```python
from build123d import *

# Parameters (mm, degrees)
SKETCH1_W            = 50.8
SKETCH1_H            = 142.24
BOSS_EXTRUDE1_DEPTH  = 38.1
SKETCH8_R            = 21.43125
BOSS_EXTRUDE2_DEPTH  = 2.54
SKETCH8_5_R          = 21.43125
BOSS_EXTRUDE9_DEPTH  = 12.7
SKETCH19_W           = 12.7
SKETCH19_H           = 6.35
BOSS_EXTRUDE10_DEPTH = 6.35
BOSS_EXTRUDE11_DEPTH = 6.35
SKETCH23_R           = 3.175
BOSS_EXTRUDE12_DEPTH = 25.4
MIRROR2_COPY_1_DEPTH = 6.35


with BuildPart() as part:
    # Sketch1 → Boss-Extrude1 (new body)
    with BuildSketch(Plane.XY):
        Rectangle(SKETCH1_W, SKETCH1_H)
    extrude(amount=BOSS_EXTRUDE1_DEPTH)



with BuildPart() as body_2:
    # Sketch8 → Boss-Extrude2 (new body)
    with BuildSketch(Plane.XZ.offset(71.12)):
        with BuildLine():
            Line((-25.4, 38.1), (25.4, 38.1))
            Line((25.4, 38.1), (25.4, 59.69))
            ThreePointArc((25.4, 59.69), (0, 85.09), (-25.4, 59.69))
            Line((-25.4, 59.69), (-25.4, 38.1))
        make_face()
        with Locations((0, 59.69)):
            Circle(SKETCH8_R, mode=Mode.SUBTRACT)
        with Locations((0, 59.69)):
            Circle(SKETCH8_R)
    extrude(amount=-BOSS_EXTRUDE2_DEPTH)


with BuildPart() as part_1:
    add(part.part)

    add(body_2.part)  # Boss-Extrude9 merges body 2
    # Sketch8<5> → Boss-Extrude9 (add)
    with BuildSketch(Plane.XZ.offset(71.12)):
        with BuildLine():
            Line((25.4, 38.1), (25.4, 59.69))
            ThreePointArc((25.4, 59.69), (0, 85.09), (-25.4, 59.69))
            Line((-25.4, 59.69), (-25.4, 38.1))
            Line((-25.4, 38.1), (25.4, 38.1))
        make_face()
        with Locations((0, 59.69)):
            Circle(SKETCH8_5_R, mode=Mode.SUBTRACT)
    extrude(amount=-BOSS_EXTRUDE9_DEPTH)

    # Sketch19 → Boss-Extrude10 (add)
    with BuildSketch(Plane.ZY.offset(25.4)):
        with Locations((31.75, 28.575)):
            Rectangle(SKETCH19_W, SKETCH19_H)
        with Locations((31.75, -3.175)):
            Rectangle(SKETCH19_W, SKETCH19_H)
    boss_extrude10 = extrude(amount=BOSS_EXTRUDE10_DEPTH)

    # Sketch20 → Boss-Extrude11 (add)
    with BuildSketch(Plane.XZ.offset(6.35)):
        with BuildLine():
            Line((-31.75, 25.4), (-31.75, 38.1))
            ThreePointArc((-31.75, 38.1), (-38.1, 31.75), (-31.75, 25.4))
        make_face()
    boss_extrude11 = extrude(amount=-BOSS_EXTRUDE11_DEPTH)

    # Mirror1: Boss-Extrude11 across plane
    add(boss_extrude11.mirror(Plane(origin=(0, 12.7, 0), x_dir=(0, 0, 1), z_dir=(0, -1, 0))))

    # Sketch23 → Boss-Extrude12 (add)
    with BuildSketch(Plane.XZ.offset(-25.4)):
        with Locations((-31.75, 31.75)):
            Circle(SKETCH23_R)
    boss_extrude12 = extrude(amount=BOSS_EXTRUDE12_DEPTH)

    # Mirror2: Boss-Extrude12, Boss-Extrude11, Boss-Extrude10 across plane
    add(boss_extrude12.mirror(Plane(origin=(0, 0, 0), x_dir=(0, 0, 1), z_dir=(1, 0, 0))))
    add(boss_extrude11.mirror(Plane(origin=(0, 0, 0), x_dir=(0, 0, 1), z_dir=(1, 0, 0))))
    add(boss_extrude10.mirror(Plane(origin=(0, 0, 0), x_dir=(0, 0, 1), z_dir=(1, 0, 0))))

    # Mirror2 copy 1 sketch → Mirror2 copy 1 (add)
    with BuildSketch(Plane(origin=(0, 31.75, 0), x_dir=(-1, 0, 0), z_dir=(0, 1, 0))):
        with BuildLine():
            Line((-31.75, 25.4), (-31.75, 38.1))
            ThreePointArc((-31.75, 38.1), (-38.1, 31.75), (-31.75, 25.4))
        make_face()
    extrude(amount=-MIRROR2_COPY_1_DEPTH)


solid = part_1.part
```
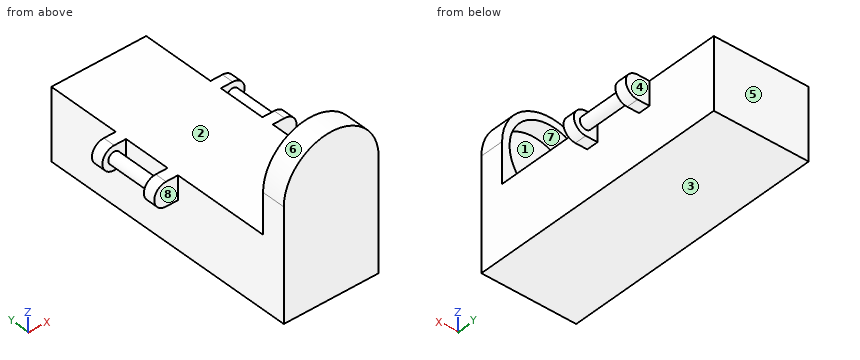
Check sheet for the modelled part. Datum: model origin and axes. Units: mm. Face numbers are marked on the shaded views. A direction names the side the tool comes from. Coordinates: 2 decimals unless noted, no trailing zeros. Write each loop counter-clockwise with the first axis right and the second up, starting at its lowest first coordinate (ties: lowest second). Pieces come first, ordered by that corner, then holes. Notation, with made-up numbers: M -27.5,79.25 L 28.5,79.25 A25 cw 28.5,104.25 Z; hole C 10.5,72.25 d1. An arc over 180 degrees is marked long. Write item = value, one per line. Start each with the question number.
1. Mould release check, pull along X, two halves, no side actions. Record for the marked faces 6, 7 and 8: pulls with the +X half, pulls with the -X half, needs draft (parallel to the pull), parting line crosses it, or undercut.
2. Thickness scan on probe 1 along X at (y, z) = (-64, 59); probe 2 along Z at (x, y) = (0, -64); probe 3 along Y at (x, z) = (29.5, 29). Record the ranges inside material, lowest first.
3. Sectioned sample at D-D (y = -45.5). Record the cut outline in (x, z).
4. Tool access check on the marked faces 1, 2, 3, 4 and 5. Record the directions out of +Z, -Z, +X, -X, +Y, -Y that give a thin tool (end or side, any length) a straight path to the whole face; none if there is none.
5. Sectioned sample at A-A (y = 15). Record the cut outline in (x, z) (3 decimals), then the cut area to 3 significant figures.
6. Sectioned sample at C-C (x = 12.5). Record the cut outline in (y, z), then the cut area to 3 significant figures.
7. Go/stop test with flat-tipped pins: pin 1 (10 mm diameter, centred on y = 12, z = 29.5, fed in from +X) (3 decimals); pin 2 (10 mm diameter, centred on x = 34, z = 31, fed in from -Y); pin 3 (19 mm diameter, centred on x = 15.5, y = 31, fed in from +Z). Record where each tip stops, or that it passes through.
8. Sectioned sample at B-B (z = 31.75). Record the cut outline in (x, y) (3 decimals), then the cut area to 3 significant figures.
The answers:
q1.face_6 = parting line crosses it
q1.face_7 = undercut
q1.face_8 = needs draft
q2.probe_1 = -25.4 to -21.42, 21.42 to 25.4
q2.probe_2 = 0 to 38.26, 81.12 to 85.09
q2.probe_3 = -6.35 to 0, 25.4 to 31.75
q3.outline = M -25.4,0 L 25.4,0 L 25.4,38.1 L -25.4,38.1 Z
q4.face_1 = +Y
q4.face_2 = +Z, +X, -X, +Y
q4.face_3 = -Z, +X, -X, +Y, -Y
q4.face_4 = +Z, -Z, +X, +Y
q4.face_5 = +Z, -Z, +X, -X, +Y
q5.outline = C -31.75,31.75 d6.35; M -25.4,0 L 25.4,0 L 25.4,38.1 L -25.4,38.1 Z; C 31.75,31.75 d6.35
q5.area = 2,000 mm²
q6.outline = M -71.12,0 L 71.12,0 L 71.12,38.1 L -58.42,38.1 L -58.42,42.28 L -68.58,42.28 L -68.58,77.1 L -58.42,77.1 L -58.42,81.8 L -71.12,81.8 Z
q6.area = 5,620 mm²
q7.pin_1 = 34.925
q7.pin_2 = -6.35
q7.pin_3 = 38.1
q8.outline = M -38.1,-6.35 L -25.4,-6.35 L -25.4,-71.12 L 25.4,-71.12 L 25.4,-6.35 L 38.1,-6.35 L 38.1,0 L 34.925,0 L 34.925,25.4 L 38.1,25.4 L 38.1,31.75 L 25.4,31.75 L 25.4,71.12 L -25.4,71.12 L -25.4,31.75 L -38.1,31.75 L -38.1,25.4 L -34.925,25.4 L -34.925,0 L -38.1,0 Z; hole M -28.575,0 L -25.4,0 L -25.4,25.4 L -28.575,25.4 Z; hole M 25.4,0 L 28.575,0 L 28.575,25.4 L 25.4,25.4 Z
q8.area = 7,870 mm²
